Source: three-view drawing plus pictorial views. Frame: mm from the lowest corner of the part. A direction names the side the tool comes from. Give positions to 0.01 mm unless a question says otherwise; leave off trailing zeros. Loops run counter-clockwise (first coordinate to the right, second up) from the corner with the lowest first, then second, coordinate; pieces in that order, holes last.
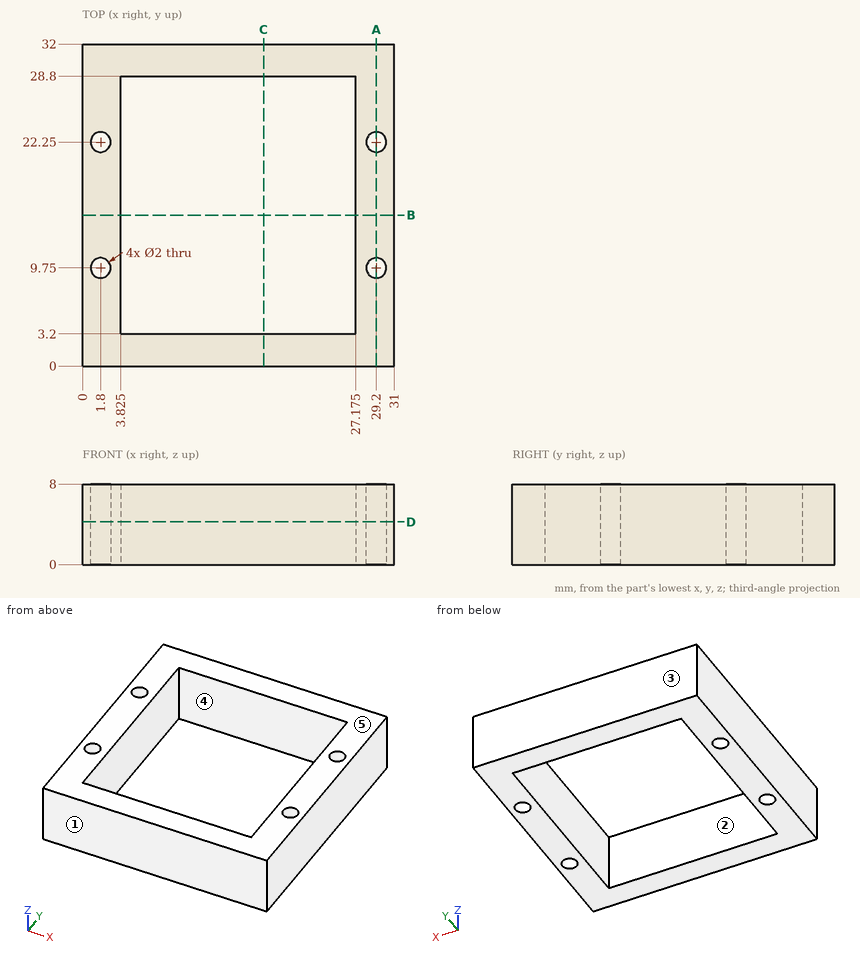
(1) Ray query, probe 1 along Y at (x, z) = (29.2, 3.25); probe 2 along Y at (x, z) = (7.5, 5.25); probe 3 along X at (y, z) = (3.5, 2.75) (3 decimals). Return the intervals inside material, ascending.
Values follow:
probe 1: y = 0 to 8.75, 10.75 to 21.25, 23.25 to 32
probe 2: y = 0 to 3.2, 28.8 to 32
probe 3: x = 0 to 3.825, 27.175 to 31
(2) Cut plane D-D (z = 4.25). Return the cut outline in (x, y) (3 decimals).
Values follow:
outline: (0, 0) - (31, 0) - (31, 32) - (0, 32) - close; hole circle Ø2 at (1.8, 9.75); hole circle Ø2 at (1.8, 22.25); hole (3.825, 3.2) - (27.175, 3.2) - (27.175, 28.8) - (3.825, 28.8) - close; hole circle Ø2 at (29.2, 9.75); hole circle Ø2 at (29.2, 22.25)
(3) Cut plane B-B (y = 15). Return the cut outline in (x, z) (3 decimals), and give its area (3 significant figures).
Values follow:
outline: (0, 0) - (3.825, 0) - (3.825, 8) - (0, 8) - close; (27.175, 0) - (31, 0) - (31, 8) - (27.175, 8) - close
area: 61.2 mm2
(4) Pin query (flat end, axial travel): pin 1 Ø4 at (x, z) = (7, 5) entering from -Y. Return the tip coordinate at first contact, or that it passes through.
Values follow:
pin 1: stops at y = 0
(5) Cut plane C-C (x = 18). Return the cut outline in (y, z), and give its area (3 significant figures).
Values follow:
outline: (0, 0) - (3.2, 0) - (3.2, 8) - (0, 8) - close; (28.8, 0) - (32, 0) - (32, 8) - (28.8, 8) - close
area: 51.2 mm2
(6) Cut plane A-A (x = 29.2). Return the cut outline in (y, z), and give its area (3 significant figures).
Values follow:
outline: (0, 0) - (8.75, 0) - (8.75, 8) - (0, 8) - close; (10.75, 0) - (21.25, 0) - (21.25, 8) - (10.75, 8) - close; (23.25, 0) - (32, 0) - (32, 8) - (23.25, 8) - close
area: 224 mm2
(7) Mould query, pull axis Y, two halves, no side actions, for the marked faces 1, 2 and 3. Classes: +Y half, -Y half, draft (parallel to the pull), parting line (faces both ways), or undercut.
Values follow:
face 1: -Y half
face 2: undercut
face 3: +Y half
(8) Reachability of the marked faces 4 and 5 from +Z, -Z, +X, -X, +Y, -Y: full face, straight path, thin tool, end or side. Return the list, or none.
Values follow:
face 4: +Z, -Z
face 5: +Z, +X, -X, +Y, -Y
